from build123d import *

# Parameters (mm, degrees)
EXTRUDE_1_DEPTH     = 1
SKETCH_2_R          = 1.5
CUT_EXTRUDE_1_DEPTH = 10
CHAMFER_1_SIZE      = 1


with BuildPart() as part:
    # Эскиз1 → Бобышка-Вытянуть1 (new body)
    with BuildSketch(Plane(origin=(0, 0, 0), x_dir=(1, 0, 0), z_dir=(0, 1, 0))):
        Polygon((15, -26), (15, -48), (-48.959081244, -48), (-48.959081244, 48), (15, 48), (15, 26), (50, 26), (50, -26), align=None)
    extrude(amount=EXTRUDE_1_DEPTH)

    # Эскиз2 → Вырез-Вытянуть1 (cut)
    with BuildSketch(Plane(origin=(0, 1, 0), x_dir=(1, 0, 0), z_dir=(0, 1, 0))):
        with Locations(Location((46.25, -14.4, 0), (0, 0, 270))):
            Circle(SKETCH_2_R)
        with Locations(Location((18.75, -14.4, 0), (0, 0, 270))):
            Circle(SKETCH_2_R)
        with Locations(Location((18.75, -4.4, 0), (0, 0, 270))):
            Circle(SKETCH_2_R)
        with Locations(Location((46.25, -4.4, 0), (0, 0, 270))):
            Circle(SKETCH_2_R)
        with Locations(Location((18.75, 5.6, 0), (0, 0, 270))):
            Circle(SKETCH_2_R)
        with Locations(Location((46.25, 5.6, 0), (0, 0, 270))):
            Circle(SKETCH_2_R)
        with Locations(Location((18.75, 15.6, 0), (0, 0, 270))):
            Circle(SKETCH_2_R)
        with Locations(Location((46.25, 15.6, 0), (0, 0, 270))):
            Circle(SKETCH_2_R)
    extrude(amount=-CUT_EXTRUDE_1_DEPTH, mode=Mode.SUBTRACT)

    # Фаска1
    chamfer_1_edges = [part.edges().sort_by_distance(p)[0] for p in [
        (46.25, 0, -7.1),
        (18.75, 0, 2.9),
        (46.25, 0, 2.9),
        (18.75, 0, 12.9),
        (18.75, 0, -17.1),
        (46.25, 0, -17.1),
        (18.75, 0, -7.1),
        (46.25, 0, 12.9),
    ]]
    chamfer(chamfer_1_edges, length=CHAMFER_1_SIZE - 0.0001)  # a hair under: the kernel refuses the full size


solid = part.part
Build history of the part. All positions in model axes, mm. Give positions to 0.01 mm unless a question says otherwise; leave off trailing zeros. Loops run counter-clockwise (first coordinate to the right, second up) from the corner with the lowest first, then second, coordinate; pieces in that order, holes last. Notation, with made-up numbers: (12.5, 76) - (60.5, 76) arc R25 cw to (60.5, 99) - close; hole circle Ø3 at (-15.5, -15.75). An arc over 180 degrees is marked (long way). Write item = value, one per line. Start each with the question number.
1) Drop flat-ended pins along their axis: pin 1 Ø4 at (x, z) = (18.75, -5.6) entering from -Y; pin 2 Ø3.5 at (x, z) = (18.75, -15.6) entering from -Y. Give the stop position or say it passes through.
2) Band-saw the part on A-A on z = 14.4. Count the separate pieces of the cut face and the enclosed holes in it, plus the area to 3 significant figures.
3) Band-saw the part on C-C on x = 35.5. Give the cut face in (y, z).
4) Probe probe 1 along Z at (x, y) = (18.5, 0.3); probe 2 along X at (y, z) = (0.4, -40.5); probe 3 along Z at (x, y) = (43, 0.55). List the from-to ranges inside material, lowest first. Write a range as from..to.
5) Band-saw the part on D-D on z = 35. Give the cut face in (x, y).
Final values:
q1.pin_1 = 0.5
q1.pin_2 = 0.75
q2.separate_pieces = 3
q2.enclosed_holes = 0
q2.area = 91.0 mm²
q3.outline = (0, -26) - (1, -26) - (1, 26) - (0, 26) - close
q4.probe_1 = -26..-17.79, -13.41..-7.79, -3.41..2.21, 6.59..12.21, 16.59..26
q4.probe_2 = -48.96..15
q4.probe_3 = -26..26
q5.outline = (-48.96, 0) - (15, 0) - (15, 1) - (-48.96, 1) - close
